Build history of the part. All positions in model axes, mm. Round coordinates to 2 decimals unless told otherwise and drop trailing zeros. Loops run counter-clockwise (first coordinate to the right, second up) from the corner with the lowest first, then second, coordinate; pieces in that order, holes last. Notation, with made-up numbers: (30.25, -13) -> (65.25, -13) arc R19 ccw to (65.25, -5) -> close; hole circle Ø2 at (63, -29.75). An arc over 180 degrees is marked (long way). Put each result on its own line as item: value. Start each with the question number.
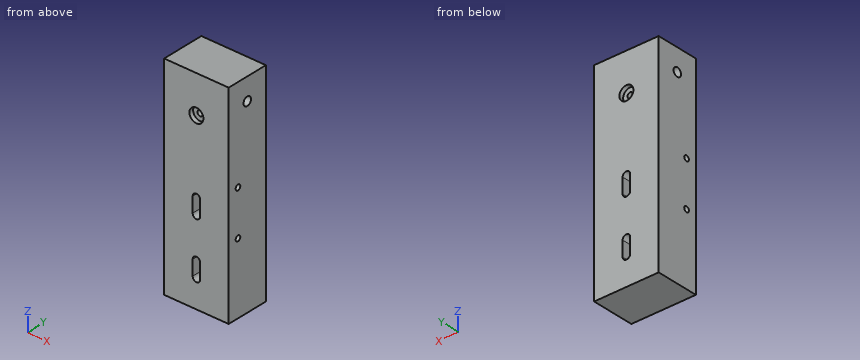
Autodesk Fusion 360 part; units mm, degrees
sketch "Skizze1" plane through (0, 0, 0) normal (0, 0, 1) x (1, 0, 0)
  line L0 (30, 20) -> (-30, 20)
  line L1 (-30, 20) -> (-30, -20)
  line L2 (-30, -20) -> (30, -20)
  line L3 (30, -20) -> (30, 20)
  line L4 (30, 20) -> (-30, -20) construction
  line L5 (-30, 20) -> (30, -20) construction
  dimension "d2" = 60
  dimension "d3" = 40
extrude "Extrusion1" add sketch "Skizze1" along normal blind 195
sketch "Skizze3" plane through (0, -20, 0) normal (0, -1, 0) x (1, 0, 0)
  line L0 (-30, 0) -> (30, 0)
  line L1 (30, 0) -> (30, 195)
  line L2 (30, 195) -> (-30, 195)
  line L3 (-30, 195) -> (-30, 0)
  line L4 (-3.5, 40) -> (-3.5, 26)
  arc A0 (-3.5, 26) -> (3.5, 26) centre (0, 26) ccw
  line L5 (3.5, 26) -> (3.5, 40)
  arc A1 (3.5, 40) -> (-3.5, 40) centre (0, 40) ccw
  line L6 (0, 40) -> (0, 26) construction
  line L7 (-3.5, 92) -> (-3.5, 78)
  arc A2 (-3.5, 78) -> (3.5, 78) centre (0, 78) ccw
  line L8 (3.5, 78) -> (3.5, 92)
  arc A3 (3.5, 92) -> (-3.5, 92) centre (0, 92) ccw
  line L9 (0, 92) -> (0, 78) construction
  point P0 (0, 195)
  dimension "d6" = 14
  dimension "d7" = 7
  dimension "d8" = 14
  dimension "d9" = 7
extrude "Extrusion2" cut sketch "Skizze3" against normal blind 40 contours L4 A0 L5 A1 | L7 A2 L8 A3
sketch "Skizze4" plane through (30, 0, 0) normal (1, 0, 0) x (0, 1, 0)
  line L0 (-20, 0) -> (20, 0)
  line L1 (20, 0) -> (20, 195)
  line L2 (20, 195) -> (-20, 195)
  line L3 (-20, 195) -> (-20, 0)
  circle A0 centre (0, 174.5) radius 4
  dimension "d12" = 8
extrude "Extrusion3" cut sketch "Skizze4" against normal blind 60 contours A0
sketch "Skizze6" plane through (0, 0, 0) normal (0, 1, 0) x (1, 0, 0)
sketch "Skizze7" plane through (0, 20, 0) normal (0, 1, 0) x (-1, 0, 0)
  line L0 (3.5, 40) -> (3.5, 26)
  arc A0 (-3.5, 26) -> (3.5, 26) centre (0, 26) ccw
  line L1 (-3.5, 26) -> (-3.5, 40)
  arc A1 (3.5, 40) -> (-3.5, 40) centre (0, 40) ccw
  line L2 (3.5, 92) -> (3.5, 78)
  arc A2 (-3.5, 78) -> (3.5, 78) centre (0, 78) ccw
  line L3 (-3.5, 78) -> (-3.5, 92)
  arc A3 (3.5, 92) -> (-3.5, 92) centre (0, 92) ccw
  line L4 (-30, 0) -> (30, 0)
  line L5 (30, 0) -> (30, 195)
  line L6 (30, 195) -> (-30, 195)
  line L7 (-30, 195) -> (-30, 0)
  circle A4 centre (0, 160) radius 2.5
  dimension "d17" = 5
extrude "Extrusion4" cut sketch "Skizze7" against normal blind 40 contours A4
sketch "Skizze9" plane through (30, 0, 0) normal (1, 0, 0) x (0, 1, 0)
  circle A0 centre (0, 174.5) radius 4
  line L0 (-20, 0) -> (20, 0)
  line L1 (20, 0) -> (20, 195)
  line L2 (20, 195) -> (-20, 195)
  line L3 (-20, 195) -> (-20, 0)
  circle A1 centre (-10, 108) radius 2.5
  circle A2 centre (-10, 66) radius 2.5
  dimension "d23" = 5
  dimension "d24" = 5
extrude "Extrusion6" cut sketch "Skizze9" against normal blind 80 contours A1 | A2
sketch "Skizze10" plane through (0, 20, 0) normal (0, 1, 0) x (-1, 0, 0)
  circle A0 centre (0, 160) radius 2.5
  line L0 (3.5, 40) -> (3.5, 26)
  arc A1 (-3.5, 26) -> (3.5, 26) centre (0, 26) ccw
  line L1 (-3.5, 26) -> (-3.5, 40)
  arc A2 (3.5, 40) -> (-3.5, 40) centre (0, 40) ccw
  line L2 (3.5, 92) -> (3.5, 78)
  arc A3 (-3.5, 78) -> (3.5, 78) centre (0, 78) ccw
  line L3 (-3.5, 78) -> (-3.5, 92)
  arc A4 (3.5, 92) -> (-3.5, 92) centre (0, 92) ccw
  line L4 (-30, 0) -> (30, 0)
  line L5 (30, 0) -> (30, 195)
  line L6 (30, 195) -> (-30, 195)
  line L7 (-30, 195) -> (-30, 0)
  circle A5 centre (0, 160) radius 6.5
  dimension "d27" = 13
extrude "Extrusion7" cut sketch "Skizze10" against normal blind 4 contours A5
sketch "Skizze11" plane through (0, -20, 0) normal (0, -1, 0) x (1, 0, 0)
  circle A0 centre (0, 160) radius 2.5
  line L0 (-3.5, 26) -> (-3.5, 40)
  arc A1 (3.5, 40) -> (-3.5, 40) centre (0, 40) ccw
  line L1 (3.5, 40) -> (3.5, 26)
  arc A2 (-3.5, 26) -> (3.5, 26) centre (0, 26) ccw
  line L2 (-3.5, 78) -> (-3.5, 92)
  arc A3 (3.5, 92) -> (-3.5, 92) centre (0, 92) ccw
  line L3 (3.5, 92) -> (3.5, 78)
  arc A4 (-3.5, 78) -> (3.5, 78) centre (0, 78) ccw
  line L4 (-30, 0) -> (30, 0)
  line L5 (30, 0) -> (30, 195)
  line L6 (30, 195) -> (-30, 195)
  line L7 (-30, 195) -> (-30, 0)
  circle A5 centre (0, 160) radius 6.5
  dimension "d30" = 13
extrude "Extrusion8" cut sketch "Skizze11" against normal blind 4 contours A5
Item 1: Cut at A-A on y = -10. Write the cut outline in (x, z).
Item 2: Wall check: line 1 (Z direction, x = 16.5, y = -10); line 2 (X direction, y = 8.5, z = 160); line 3 (Z direction, x = 1, y = 7). Give the ranges that are in metal, low to high. Write a range as from..to.
Item 3: Drop flat-ended pins along their axis: pin 1 (4 mm diameter, centred on x = 16.5, y = -11.5, fed in from -Z); pin 2 (4 mm diameter, centred on x = 0.5, z = 162, fed in from +Y); pin 3 (4 mm diameter, centred on x = 2.5, z = 161.5, fed in from -Y). Give the stop position or say it passes through.
Item 4: Cut at B-B on z = 174.5. Write the cut outline in (x, y), then the cut area to 3 significant figures.
Item 5: Cut at D-D on z = 66. Write the cut outline in (x, y).
Item 6: Cut at C-C on y = 10.5. Write the cut outline in (x, z).
Ans:
1. outline: (-30, 0) -> (30, 0) -> (30, 63.5) -> (-30, 63.5) -> close; (-30, 68.5) -> (30, 68.5) -> (30, 105.5) -> (-30, 105.5) -> close; (-30, 110.5) -> (30, 110.5) -> (30, 195) -> (-30, 195) -> close; hole (-3.5, 26) arc R3.5 ccw to (3.5, 26) -> (3.5, 40) arc R3.5 ccw to (-3.5, 40) -> close; hole (-3.5, 78) arc R3.5 ccw to (3.5, 78) -> (3.5, 92) arc R3.5 ccw to (-3.5, 92) -> close; hole circle Ø5 at (0, 160)
2. line 1: z = 0..63.5, 68.5..105.5, 110.5..195
2. line 2: x = -30..-2.5, 2.5..30
2. line 3: z = 0..22.65, 43.35..74.65, 95.35..157.71, 162.29..195
3. pin 1: stops at z = 0
3. pin 2: stops at y = 16
3. pin 3: stops at y = -16
4. outline: (-30, -20) -> (30, -20) -> (30, -4) -> (-30, -4) -> close; (-30, 4) -> (30, 4) -> (30, 20) -> (-30, 20) -> close
4. area: 1,920 mm2
5. outline: (-30, -20) -> (30, -20) -> (30, -12.5) -> (-30, -12.5) -> close; (-30, -7.5) -> (30, -7.5) -> (30, 20) -> (-30, 20) -> close
6. outline: (-30, 0) -> (30, 0) -> (30, 195) -> (-30, 195) -> close; hole (-3.5, 26) arc R3.5 ccw to (3.5, 26) -> (3.5, 40) arc R3.5 ccw to (-3.5, 40) -> close; hole (-3.5, 78) arc R3.5 ccw to (3.5, 78) -> (3.5, 92) arc R3.5 ccw to (-3.5, 92) -> close; hole circle Ø5 at (0, 160)
